from build123d import *

# Parameters (mm, degrees)
F6_R      = 1.5
F7_DEPTH  = 29.2
F4_R      = 1.5
F8_DEPTH  = 2.1
F1_W      = 3.3
F1_H      = 10
F0_W      = 3.3
F0_H      = 10
F9_DEPTH  = 6.1
F10_DEPTH = 40.9


with BuildPart() as f7:
    # F6 (on offset) → F7 (new body)
    with BuildSketch(Plane.XY.offset(2.1)):
        Polygon((33.1796569254, 61.95), (2.5, 61.95), (-26.3796569254, 61.95), (-41.05, 39.6376911413), (-41.05, -3.3), (47.85, -3.3), (47.85, 39.6376911413), align=None)
        Polygon((44.55, 29.97), (44.55, 7.15), (44.55, 0), (37.4, 0), (-30.6, 0), (-37.75, 0), (-37.75, 7.15), (-37.75, 29.97), (-37.75, 38.65), (-35.7847248185, 41.6390116829), (-27.896317712, 53.6365890312), (-24.6, 58.65), (-18.6, 58.65), (3.4, 58.65), (25.4, 58.65), (31.4, 58.65), (34.696317712, 53.6365890312), (42.5847248185, 41.6390116829), (44.55, 38.65), (44.55, 36.9490727423), align=None, mode=Mode.SUBTRACT)
        with BuildLine():
            ThreePointArc((42.5847248185, 41.6390116829), (38.6333256766, 34.9735237327), (44.55, 29.97))
            Line((44.55, 29.97), (44.55, 36.9490727423))
            Line((44.55, 36.9490727423), (44.55, 38.65))
            Line((44.55, 38.65), (42.5847248185, 41.6390116829))
        make_face()
        with Locations((41.87, 35.97)):
            Circle(F6_R, mode=Mode.SUBTRACT)
        with BuildLine():
            Line((-37.75, 38.65), (-37.75, 29.97))
            ThreePointArc((-37.75, 29.97), (-31.8333256766, 34.9735237327), (-35.7847248185, 41.6390116829))
            Line((-35.7847248185, 41.6390116829), (-37.75, 38.65))
        make_face()
        with Locations((-35.07, 35.97)):
            Circle(F6_R, mode=Mode.SUBTRACT)
        with BuildLine():
            Line((44.55, 0), (44.55, 7.15))
            ThreePointArc((44.55, 7.15), (39.4941865145, 5.0558134855), (37.4, 0))
            Line((37.4, 0), (44.55, 0))
        make_face()
        with Locations((41.87, 2.68)):
            Circle(F6_R, mode=Mode.SUBTRACT)
        with BuildLine():
            Line((-37.75, 0), (-30.6, 0))
            ThreePointArc((-30.6, 0), (-32.6941865145, 5.0558134855), (-37.75, 7.15))
            Line((-37.75, 7.15), (-37.75, 0))
        make_face()
        with Locations((-35.07, 2.68)):
            Circle(F6_R, mode=Mode.SUBTRACT)
        with BuildLine():
            ThreePointArc((25.4, 58.65), (28.5520100309, 53.3690007446), (34.696317712, 53.6365890312))
            Line((34.696317712, 53.6365890312), (31.4, 58.65))
            Line((31.4, 58.65), (25.4, 58.65))
        make_face()
        with Locations((30.3835309261, 55.8274496246)):
            Circle(F6_R, mode=Mode.SUBTRACT)
        with BuildLine():
            Line((-24.6, 58.65), (-27.896317712, 53.6365890312))
            ThreePointArc((-27.896317712, 53.6365890312), (-21.7520100309, 53.3690007446), (-18.6, 58.65))
            Line((-18.6, 58.65), (-24.6, 58.65))
        make_face()
        with Locations((-23.5835309261, 55.8274496246)):
            Circle(F6_R, mode=Mode.SUBTRACT)
    extrude(amount=F7_DEPTH)



with BuildPart() as f8:
    # F4 (on Top) → F8 (new body)
    with BuildSketch(Plane.XY):
        Polygon((33.1796569254, 61.95), (2.5, 61.95), (-26.3796569254, 61.95), (-41.05, 39.6376911413), (-41.05, -3.3), (47.85, -3.3), (47.85, 39.6376911413), align=None)
        with BuildLine():
            Line((44.55, 7.15), (44.55, 0))
            Line((44.55, 0), (37.4, 0))
            Line((37.4, 0), (-30.6, 0))
            Line((-30.6, 0), (-37.75, 0))
            Line((-37.75, 0), (-37.75, 7.15))
            Line((-37.75, 7.15), (-37.75, 29.97))
            Line((-37.75, 29.97), (-37.75, 38.65))
            Line((-37.75, 38.65), (-35.7847248185, 41.6390116829))
            Line((-35.7847248185, 41.6390116829), (-27.896317712, 53.6365890312))
            Line((-27.896317712, 53.6365890312), (-24.6, 58.65))
            Line((-24.6, 58.65), (-18.6, 58.65))
            Line((-18.6, 58.65), (3.4, 58.65))
            Line((3.4, 58.65), (25.4, 58.65))
            Line((25.4, 58.65), (31.4, 58.65))
            Line((31.4, 58.65), (34.696317712, 53.6365890312))
            Line((34.696317712, 53.6365890312), (42.5847248185, 41.6390116829))
            ThreePointArc((42.5847248185, 41.6390116829), (38.6333256766, 34.9735237327), (44.55, 29.97))
            Line((44.55, 29.97), (44.55, 7.15))
        make_face(mode=Mode.SUBTRACT)
        with BuildLine():
            Line((-30.6, 0), (37.4, 0))
            ThreePointArc((37.4, 0), (39.4941865145, 5.0558134855), (44.55, 7.15))
            Line((44.55, 7.15), (44.55, 29.97))
            ThreePointArc((44.55, 29.97), (38.6333256766, 34.9735237327), (42.5847248185, 41.6390116829))
            Line((42.5847248185, 41.6390116829), (34.696317712, 53.6365890312))
            ThreePointArc((34.696317712, 53.6365890312), (28.5520100309, 53.3690007446), (25.4, 58.65))
            Line((25.4, 58.65), (3.4, 58.65))
            Line((3.4, 58.65), (-18.6, 58.65))
            ThreePointArc((-18.6, 58.65), (-21.7520100309, 53.3690007446), (-27.896317712, 53.6365890312))
            Line((-27.896317712, 53.6365890312), (-35.7847248185, 41.6390116829))
            ThreePointArc((-35.7847248185, 41.6390116829), (-31.8333256766, 34.9735237327), (-37.75, 29.97))
            Line((-37.75, 29.97), (-37.75, 7.15))
            ThreePointArc((-37.75, 7.15), (-32.6941865145, 5.0558134855), (-30.6, 0))
        make_face()
        with BuildLine():
            Line((-37.75, 38.65), (-37.75, 29.97))
            ThreePointArc((-37.75, 29.97), (-31.8333256766, 34.9735237327), (-35.7847248185, 41.6390116829))
            Line((-35.7847248185, 41.6390116829), (-37.75, 38.65))
        make_face()
        with BuildLine():
            Line((-37.75, 0), (-30.6, 0))
            ThreePointArc((-30.6, 0), (-32.6941865145, 5.0558134855), (-37.75, 7.15))
            Line((-37.75, 7.15), (-37.75, 0))
        make_face()
        with BuildLine():
            Line((37.4, 0), (44.55, 0))
            Line((44.55, 0), (44.55, 7.15))
            ThreePointArc((44.55, 7.15), (39.4941865145, 5.0558134855), (37.4, 0))
        make_face()
        with BuildLine():
            ThreePointArc((25.4, 58.65), (28.5520100309, 53.3690007446), (34.696317712, 53.6365890312))
            Line((34.696317712, 53.6365890312), (31.4, 58.65))
            Line((31.4, 58.65), (25.4, 58.65))
        make_face()
        with Locations((30.3835309261, 55.8274496246)):
            Circle(F4_R, mode=Mode.SUBTRACT)
        with BuildLine():
            Line((-24.6, 58.65), (-27.896317712, 53.6365890312))
            ThreePointArc((-27.896317712, 53.6365890312), (-21.7520100309, 53.3690007446), (-18.6, 58.65))
            Line((-18.6, 58.65), (-24.6, 58.65))
        make_face()
        with Locations((-23.5835309261, 55.8274496246)):
            Circle(F4_R, mode=Mode.SUBTRACT)
        with Locations((30.3835309261, 55.8274496246)):
            Circle(F4_R)
        with Locations((-23.5835309261, 55.8274496246)):
            Circle(F4_R)
    extrude(amount=F8_DEPTH)


with BuildPart() as f7_1:
    add(f7.part)

    add(f8.part)  # F9 merges F8
    # F1 (on Top) + F0 (on Top) → F9 (join)
    with BuildSketch(Plane.XY):
        with Locations((-29.25, 40.5)):
            Rectangle(F1_W, F1_H)
        Polygon((-30.9, 45.5), (-27.6, 45.5), (-22.9, 45.5), (-22.9, 48.8), (-30.9, 48.8), align=None)
        with Locations((-29.25, 5)):
            Rectangle(F1_W, F1_H)
        with Locations((-5.95, 5)):
            Rectangle(F1_W, F1_H)
        with Locations((-5.95, 40.5)):
            Rectangle(F1_W, F1_H)
        Polygon((-12.3, 45.5), (-7.6, 45.5), (-4.3, 45.5), (-4.3, 48.8), (-12.3, 48.8), align=None)
    with BuildSketch(Plane.XY):
        with Locations((-1.65, 5)):
            Rectangle(F0_W, F0_H)
        with Locations((2.93, 43.45)):
            Rectangle(F0_W, F0_H)
        Polygon((1.28, 48.45), (4.58, 48.45), (14.58, 48.45), (14.58, 51.75), (1.28, 51.75), align=None)
        Polygon((19.52, 51.75), (19.52, 48.45), (29.52, 48.45), (32.82, 48.45), (32.82, 51.75), align=None)
        with Locations((31.17, 43.45)):
            Rectangle(F0_W, F0_H)
        with Locations((35.75, 5)):
            Rectangle(F0_W, F0_H)
    extrude(amount=F9_DEPTH)

    # F6 (on offset) → F10 (join)
    with BuildSketch(Plane.XY.offset(2.1)):
        Polygon((33.1796569254, 61.95), (2.5, 61.95), (-26.3796569254, 61.95), (-41.05, 39.6376911413), (-41.05, -3.3), (47.85, -3.3), (47.85, 39.6376911413), align=None)
        Polygon((44.55, 29.97), (44.55, 7.15), (44.55, 0), (37.4, 0), (-30.6, 0), (-37.75, 0), (-37.75, 7.15), (-37.75, 29.97), (-37.75, 38.65), (-35.7847248185, 41.6390116829), (-27.896317712, 53.6365890312), (-24.6, 58.65), (-18.6, 58.65), (3.4, 58.65), (25.4, 58.65), (31.4, 58.65), (34.696317712, 53.6365890312), (42.5847248185, 41.6390116829), (44.55, 38.65), (44.55, 36.9490727423), align=None, mode=Mode.SUBTRACT)
    extrude(amount=F10_DEPTH)


solid = f7_1.part
The listing builds one solid part. Answer for the finished solid, in the listing's coordinates (mm). Coordinates: 2 decimals unless noted, no trailing zeros. Write each loop counter-clockwise with the first axis right and the second up, starting at its lowest first coordinate (ties: lowest second). Pieces come first, ordered by that corner, then holes. Notation, with made-up numbers: M 80.25,-15.75 L 130.25,-15.75 A3 cw 130.25,-11.75 Z; hole C 17.5,23 d8. An arc over 180 degrees is marked long. Put each result on its own line as item: value. Start each with the question number.
1. A cutting plane is placed at D-D on z = 17.5. Write down the section's boundary in (x, y), then the cut area to 3 significant figures.
2. A cutting plane is placed at B-B on z = 32.5. Write down the section's boundary in (x, y).
3. Flat-ended cylindrical pins translate along their axes: P1, Ø4, axis at x = 24.5, y = 46, coming from the +Z side; P2, Ø1, axis at x = -2, y = 3, coming from the +Z side; P3, Ø1.6, axis at y = 51, z = 4.5, coming from the -X side. Find the tip coordinate at first contact, or state that the pin passes through.
4. A cutting plane is placed at A-A on x = 10.5. Write down the section's boundary in (y, z), then the cut area to 3 significant figures.
5. For a pull along Y with two mould halves and no side action, classify faces 1 (the flat face through (47.85, 18, 21)), 2 (the flat face through (8, 51.75, 4)), 3 (the flat face through (40.618, 50.638, 21.199)) as pulls with the +Y half, pulls with the -Y half, needs draft (parallel to the pull), parting line crosses it, or undercut.
6. A cutting plane is placed at C-C on y = 47. Write down the section's boundary in (x, z).
7. Consider line 1 (Y direction, x = 2.5, z = 7); line 2 (X direction, y = 13, z = 12.5); line 3 (Y direction, x = -2, z = 6). Determine where each line is inside the solid, lowest interval first. Write a range as from..to.
Resolved:
1. outline: M -41.05,-3.3 L 47.85,-3.3 L 47.85,39.64 L 33.18,61.95 L -26.38,61.95 L -41.05,39.64 Z; hole M -37.75,7.15 A7.15 cw -30.6,0 L 37.4,0 A7.15 cw 44.55,7.15 L 44.55,29.97 A6 cw 42.58,41.64 L 34.7,53.64 A6 cw 25.4,58.65 L -18.6,58.65 A6 cw -27.9,53.64 L -35.78,41.64 A6 cw -37.75,29.97 Z; hole C -35.07,2.68 d3; hole C -35.07,35.97 d3; hole C -23.58,55.83 d3; hole C 30.38,55.83 d3; hole C 41.87,2.68 d3; hole C 41.87,35.97 d3
1. area: 1,130 mm2
2. outline: M -41.05,-3.3 L 47.85,-3.3 L 47.85,39.64 L 33.18,61.95 L -26.38,61.95 L -41.05,39.64 Z; hole M -37.75,0 L 44.55,0 L 44.55,38.65 L 31.4,58.65 L -24.6,58.65 L -37.75,38.65 Z
3. P1: stops at z = 2.1
3. P2: stops at z = 6.1
3. P3: stops at x = -34.11
4. outline: M -3.3,0 L 61.95,0 L 61.95,43 L 58.65,43 L 58.65,2.1 L 51.75,2.1 L 51.75,6.1 L 48.45,6.1 L 48.45,2.1 L 0,2.1 L 0,43 L -3.3,43 Z
4. area: 420 mm2
5. face 1: needs draft
5. face 2: undercut
5. face 3: pulls with the +Y half
6. outline: M -36.21,0 L 43.01,0 L 43.01,43 L 39.06,43 L 39.06,2.1 L 32.82,2.1 L 32.82,6.1 L 29.52,6.1 L 29.52,2.1 L 4.58,2.1 L 4.58,6.1 L 1.28,6.1 L 1.28,2.1 L -4.3,2.1 L -4.3,6.1 L -12.3,6.1 L -12.3,2.1 L -22.9,2.1 L -22.9,6.1 L -30.9,6.1 L -30.9,2.1 L -32.26,2.1 L -32.26,43 L -36.21,43 Z
7. line 1: y = -3.3..0, 58.65..61.95
7. line 2: x = -41.05..-37.75, 44.55..47.85
7. line 3: y = -3.3..10, 58.65..61.95
